Source: CAD feature listing. Evaluate the final solid. Frame: model axes, mm. Face numbers are marked on the shaded views. Give positions to 0.01 mm unless a question says otherwise; leave off trailing zeros. Loops run counter-clockwise (first coordinate to the right, second up) from the corner with the lowest first, then second, coordinate; pieces in that order, holes last. Notation, with made-up numbers: (-24.5, 43.25) - (-12.5, 43.25) arc R5 cw to (-12.5, 47.25) - close; hole circle Ø1 at (73.5, -20.5). An arc over 180 degrees is marked (long way). Put each result on its own line as item: value.
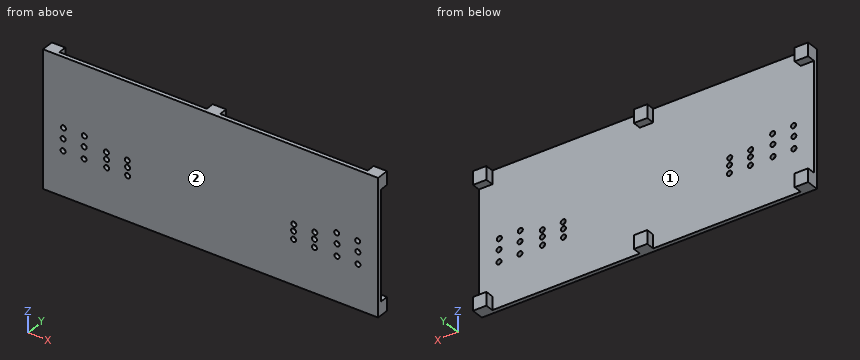
```python
from build123d import *

# Parameters (mm, degrees)
SKETCH1_W           = 100
SKETCH1_H           = 81
BOSS_EXTRUDE1_DEPTH = 2.5
SKETCH3_R           = 1.5
CUT_EXTRUDE1_DEPTH  = 108.91895107
SKETCH4_W           = 8
SKETCH4_H           = 8
SKETCH4_W_2         = 4
BOSS_EXTRUDE2_DEPTH = 5


with BuildPart() as part:
    # Sketch1 → Boss-Extrude1 (new body)
    with BuildSketch(Plane(origin=(0, 0, 0), x_dir=(1, 0, 0), z_dir=(0, 1, 0))):
        with Locations((50, 0)):
            Rectangle(SKETCH1_W, SKETCH1_H)
    boss_extrude1 = extrude(amount=-BOSS_EXTRUDE1_DEPTH)

    # Sketch3 → Cut-Extrude1 (cut, through all)
    with BuildSketch(Plane(origin=(0, 0, 0), x_dir=(1, 0, 0), z_dir=(0, 1, 0))):
        with Locations(Location((88, 14, 0), (0, 0, 270))):
            Circle(SKETCH3_R)
        with Locations(Location((62, 14, 0), (0, 0, 90))):
            Circle(SKETCH3_R)
        with Locations(Location((62.049468925, 9.152599975, 0), (0, 0, 270))):
            Circle(SKETCH3_R)
        with Locations(Location((87.950531075, 6.886550664, 0), (0, 0, 270))):
            Circle(SKETCH3_R)
        with Locations(Location((62.197499211, 5.073814511, 0), (0, 0, 270))):
            Circle(SKETCH3_R)
        with Locations(Location((87.802500789, 0.558961892, 0), (0, 0, 270))):
            Circle(SKETCH3_R)
        with Locations(Location((49.5, 14, 0), (0, 0, 270))):
            Circle(SKETCH3_R)
        with Locations(Location((75.5, 14, 0), (0, 0, 270))):
            Circle(SKETCH3_R)
        with Locations(Location((49.549468925, 9.152599975, 0), (0, 0, 270))):
            Circle(SKETCH3_R)
        with Locations(Location((75.450531075, 6.886550664, 0), (0, 0, 270))):
            Circle(SKETCH3_R)
        with Locations(Location((49.697499211, 5.073814511, 0), (0, 0, 270))):
            Circle(SKETCH3_R)
        with Locations(Location((75.302500789, 0.558961892, 0), (0, 0, 270))):
            Circle(SKETCH3_R)
    cut_extrude1 = extrude(amount=-CUT_EXTRUDE1_DEPTH, mode=Mode.SUBTRACT)

    # Sketch4 → Boss-Extrude2 (add)
    with BuildSketch(Plane(origin=(0, 0, 0), x_dir=(1, 0, 0), z_dir=(0, 1, 0))):
        with Locations((96, -36.5)):
            Rectangle(SKETCH4_W, SKETCH4_H)
        with Locations((96, 36.5)):
            Rectangle(SKETCH4_W, SKETCH4_H)
        with Locations((2, -36.5)):
            Rectangle(SKETCH4_W_2, SKETCH4_H)
        with Locations((2, 36.5)):
            Rectangle(SKETCH4_W_2, SKETCH4_H)
    boss_extrude2 = extrude(amount=BOSS_EXTRUDE2_DEPTH)

    # Mirror1: Boss-Extrude1, Cut-Extrude1, Boss-Extrude2 across plane
    add(boss_extrude1.mirror(Plane(origin=(0, 0, 0), x_dir=(0, 0, 1), z_dir=(1, 0, 0))))
    add(cut_extrude1.mirror(Plane(origin=(0, 0, 0), x_dir=(0, 0, 1), z_dir=(1, 0, 0))), mode=Mode.SUBTRACT)
    add(boss_extrude2.mirror(Plane(origin=(0, 0, 0), x_dir=(0, 0, 1), z_dir=(1, 0, 0))))


solid = part.part
```
1) Pin query (flat end, axial travel): P1, Ø4, axis at x = 87.95, z = -6.89, coming from the +Y side. Return the tip coordinate at first contact, or that it passes through.
Check result:
P1: y = 0
2) Material intervals for line 1 along X through (y, z) = (0.25, 33); line 2 along Z through (x, y) = (75.5, -1.8); line 3 along X through (y, z) = (-1.25, -5), sorted ascending. Write a range as [from, to].
Check result:
line 1: [-100, -92], [-4, 4], [92, 100]
line 2: [-40.5, -15.5], [-12.5, -8.39], [-5.39, -2.05], [0.93, 40.5]
line 3: [-100, -63.7], [-60.7, -51.2], [-48.2, 48.2], [51.2, 60.7], [63.7, 100]
3) Section query A-A, the plane y = 3. Output: boundary loops of the cut face in (x, z), plus the area to 3 significant figures.
Check result:
outline: (-100, -40.5) - (-92, -40.5) - (-92, -32.5) - (-100, -32.5) - close; (-100, 32.5) - (-92, 32.5) - (-92, 40.5) - (-100, 40.5) - close; (-4, -40.5) - (4, -40.5) - (4, -32.5) - (-4, -32.5) - close; (-4, 32.5) - (4, 32.5) - (4, 40.5) - (-4, 40.5) - close; (92, -40.5) - (100, -40.5) - (100, -32.5) - (92, -32.5) - close; (92, 32.5) - (100, 32.5) - (100, 40.5) - (92, 40.5) - close
area: 384 mm²
4) Section query C-C, the plane z = 17.5. Output: boundary loops of the cut face in (x, y).
Check result:
outline: (-100, -2.5) - (100, -2.5) - (100, 0) - (-100, 0) - close
5) Mould query, pull axis X, two halves, no side actions, for the marked faces 1 and 2. Classes: pulls with the +X half, pulls with the -X half, needs draft (parallel to the pull), parting line crosses it, or undercut.
Check result:
face 1: undercut
face 2: needs draft
6) Section query B-B, the plane x = 68. Output: boundary loops of the cut face in (y, z), plus the area to 4 significant figures.
Check result:
outline: (-2.5, -40.5) - (0, -40.5) - (0, 40.5) - (-2.5, 40.5) - close
area: 202.5 mm²
